from build123d import *

# Parameters (mm, degrees)
F0_W     = 38.677551
F0_H     = 87.183475
F1_DEPTH = 25.4
F2_R     = 10.61277
F3_DEPTH = 36.733858
F4_SIZE  = 5.08


with BuildPart() as f1:
    # F0 (on Front) → F1 (new body)
    with BuildSketch(Plane.XZ):
        with Locations((39.677791, 5.360209)):
            Rectangle(F0_W, F0_H)
    extrude(amount=F1_DEPTH)

    # F2 (on face) → F3 (join)
    with BuildSketch(Plane.XZ.offset(25.4)):
        with Locations((41.557305, 14.468271)):
            Circle(F2_R)
    extrude(amount=F3_DEPTH)

    # F4
    f4_edges = [f1.edges().sort_by_distance(p)[0] for p in [
        (20.339016, -25.4, 5.360208),
    ]]
    chamfer(f4_edges, length=F4_SIZE)


solid = f1.part
The model under review builds one solid part; all positions refer to its coordinate system, in mm. A direction names the side the tool comes from. Give positions to 0.01 mm unless a question says otherwise; leave off trailing zeros. Write each loop counter-clockwise with the first axis right and the second up, starting at its lowest first coordinate (ties: lowest second). Pieces come first, ordered by that corner, then holes.
1. For P1, Ø4, axis at x = 34, y = -52, coming from the -Z side; P2, Ø2, axis at x = 30, z = 17, coming from the -Y side; P3, Ø8, axis at x = 44.5, y = -31.5, coming from the -Z side, all flat-tipped, find the tip position at first contact; note any pin that passes through.
2. Tool access review of faces 1 (the cylindrical face through (33.135, -43.51, 8.011)), 2 (the flat face through (41, -62.134, 15)): name each direction out of +Z, -Z, +X, -X, +Y, -Y from which nothing blocks a thin tool from reaching the whole face with its end or side.
3. Wall thickness on L1, parallel to Y at x = 35, z = -28; L2, parallel to Z at x = 42, y = -39.5; L3, parallel to Z at x = 43, y = -56: over which ranges is each line inside the solid? List them lowest first.
4. Add section B-B, the plane x = 46. Write out the cut boundary in (y, z).
5. Add section C-C, the plane y = -56. Write out the cut boundary in (x, z).
6. Add section A-A, the plane z = -15. Write out the cut boundary in (x, y).
7. Add section D-D, the plane x = 51. Write out the cut boundary in (y, z), plus the area to 3 significant figures.
Worked answers:
1. P1: stops at z = 5.43
1. P2: stops at y = -25.4
1. P3: stops at z = 3.86
2. face 1: -Y
2. face 2: +Z, -Z, +X, -X, -Y
3. L1: y = -25.4 to 0
3. L2: z = 3.86 to 25.07
3. L3: z = 3.95 to 24.98
4. outline: (-62.13, 4.83) - (-25.4, 4.83) - (-25.4, -38.23) - (0, -38.23) - (0, 48.95) - (-25.4, 48.95) - (-25.4, 24.11) - (-62.13, 24.11) - close
5. outline: circle Ø21.23 at (41.56, 14.47)
6. outline: (20.34, -20.32) - (25.42, -25.4) - (59.02, -25.4) - (59.02, 0) - (20.34, 0) - close
7. outline: (-62.13, 9.62) - (-25.4, 9.62) - (-25.4, -38.23) - (0, -38.23) - (0, 48.95) - (-25.4, 48.95) - (-25.4, 19.31) - (-62.13, 19.31) - close
7. area: 2,570 mm2
